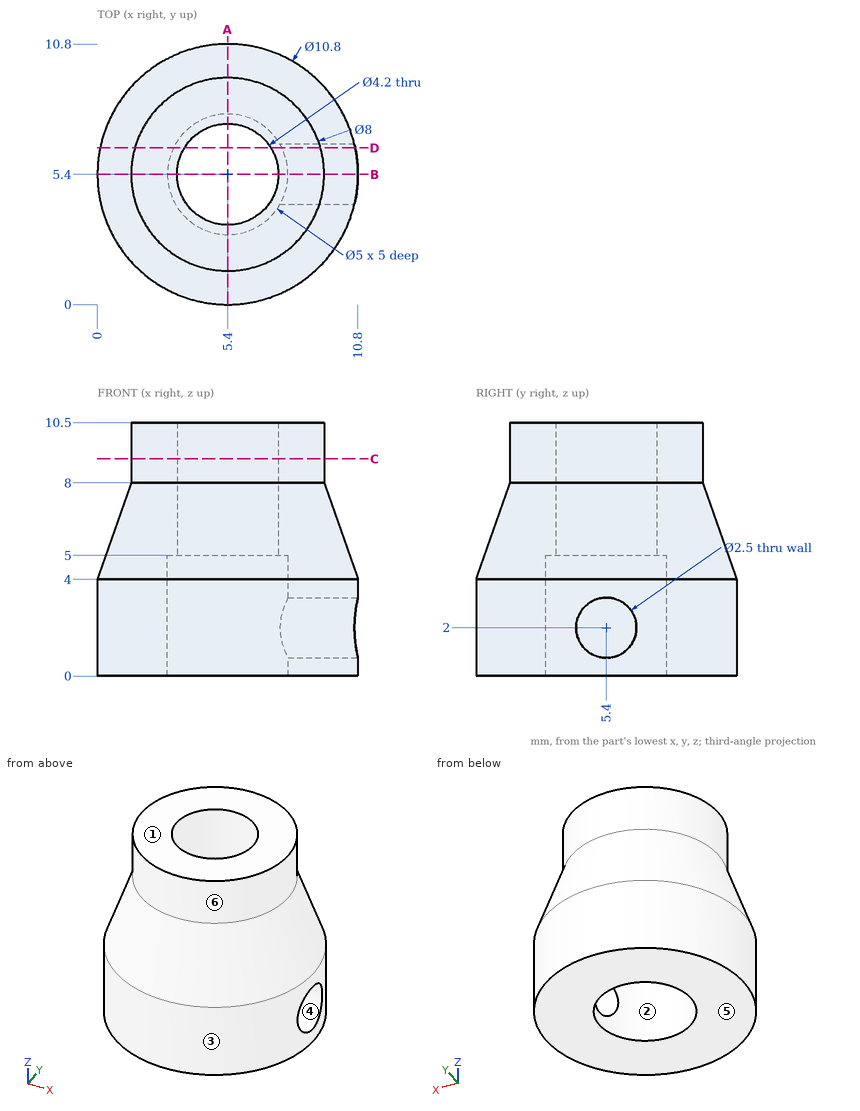
Part print with two shaded views. Sizes in mm from the minimum x, y, z corner. A direction names the side the tool comes from. Round coordinates to 2 decimals unless told otherwise and drop trailing zeros. Loops run counter-clockwise (first coordinate to the right, second up) from the corner with the lowest first, then second, coordinate; pieces in that order, holes last. Notation, with made-up numbers: (-38, 83) - (-5, 83) arc R21 ccw to (-5, 119) - close; hole circle Ø10 at (10, 67). An arc over 180 degrees is marked (long way). Put each result on its own line as item: value.
1. Slice it at C-C on z = 9. List the corners of the cut face in (x, y).
Geometry check:
outline: circle Ø8 at (5.4, 5.4); hole circle Ø4.2 at (5.4, 5.4)
2. Wall check: line 1 (Y direction, x = 5.4, z = 3.45); line 2 (X direction, y = 5.5, z = 10); line 3 (X direction, y = 5.5, z = 1.5). Give the ranges that are in metal, low to high.
Geometry check:
line 1: 0 to 2.9, 7.9 to 10.8
line 2: 1.4 to 3.3, 7.5 to 9.4
line 3: 0 to 2.9
3. Pin check, flat tips, straight feed: P1, Ø2, axis at x = 2, z = 7.5, coming from the +Y side; P2, Ø3, axis at x = 2.5, z = 3, coming from the -Y side; P3, Ø2, axis at x = 5, z = 6, coming from the +Y side. Stop position of each tip, or through.
Geometry check:
P1: y = 8.94
P2: y = 0.18
P3: y = 10.44
4. Slice it at B-B on y = 5.4. List the corners of the cut face in (x, z).
Geometry check:
outline: (0, 0) - (2.9, 0) - (2.9, 5) - (3.3, 5) - (3.3, 10.5) - (1.4, 10.5) - (1.4, 8) - (0, 4) - close; (7.5, 5) - (7.9, 5) - (7.9, 3.25) - (10.8, 3.25) - (10.8, 4) - (9.4, 8) - (9.4, 10.5) - (7.5, 10.5) - close; (7.9, 0) - (10.8, 0) - (10.8, 0.75) - (7.9, 0.75) - close
5. Slice it at D-D on y = 6.5. Give the number of separate pieces and of enclosed holes in the cut face, and give its area (3 significant figures).
Geometry check:
separate pieces: 3
enclosed holes: 0
area: 52.3 mm²
6. 3-axis set-ups, long thin cutter, end or side, ignore diameter. For the marked faces 4, 5 and 6: which of +Z, -Z, +X, -X, +Y, -Y reach the whole face in a straight line?
Geometry check:
face 4: +X
face 5: -Z, +X, -X, +Y, -Y
face 6: +Z
7. Slice it at A-A on x = 5.4. List the corners of the cut face in (y, z), and give its area (3 significant figures).
Geometry check:
outline: (0, 0) - (2.9, 0) - (2.9, 5) - (3.3, 5) - (3.3, 10.5) - (1.4, 10.5) - (1.4, 8) - (0, 4) - close; (7.5, 5) - (7.9, 5) - (7.9, 0) - (10.8, 0) - (10.8, 4) - (9.4, 8) - (9.4, 10.5) - (7.5, 10.5) - close
area: 52.7 mm²
8. Two-plate mould, pull along X, no slides. Class the marked faces 1, 2 and 3: released by +X, released by -X, zero draft, split by the parting line, or undercut.
Geometry check:
face 1: zero draft
face 2: undercut
face 3: split by the parting line
